Model file for the job. Use its own axes, mm. Give positions to 0.01 mm unless a question says otherwise; leave off trailing zeros. Order: outer loops, then holes, each group sorted by start corner. A loop starts at its lowest first (then second) coordinate and runs counter-clockwise, first axis right, second up. Notation, with made-up numbers: M 40,47 L 87,47 A24 ccw 87,57 Z; hole C 20.25,-31 d9. An arc over 180 degrees is marked long. Return JSON: item names as keys, results as strings. Group by question number.
1. Slice it at B-B on x = 13.5. List the corners of the cut face in (y, z), then the cut area to 3 significant figures.
2. Slice it at A-A on x = -18. List the corners of the cut face in (y, z), then the cut area to 3 significant figures.
3. Pin check, flat tip, straight feed: pin 1 (2 mm diameter, centred on x = -10.5, z = 4.5, fed in from -Y). Stop position of the tip, or through.
4. Wall check: probe 1 along Y at (x, z) = (-15.5, 0); probe 2 along Z at (x, y) = (-8, 12.7); probe 3 along Z at (x, y) = (-22.5, 5.75). Give the ranges that are in metal, low to high. Write a range as [from, to].
5. Two-plate mould, pull along Y, no slides. Class faces 1 (the face through (0, 25.4, 0)), 2 (the face through (0, 13, 12.7)), 3 (the face through (-6, 4, 2)), 4 (the face through (7.232, 1.229, 0.805)): released by +Y, released by -Y, zero draft, split by the parting line, or undercut.
from build123d import *

# Parameters (mm, degrees)
SKETCH1_W                         = 50.8
SKETCH1_H                         = 25.4
BOSS_EXTRUDE1_DEPTH               = 25.4
PIPE_TAP_DRILL_FOR_1_2_TAP1_D     = 17.8562
PIPE_TAP_DRILL_FOR_1_2_TAP1_DEPTH = 38.1
PIPE_TAP_DRILL_FOR_1_2_TAP1_TIP   = 5.364543693


with BuildPart() as part:
    # Sketch1 → Boss-Extrude1 (new body)
    with BuildSketch(Plane(origin=(0, 0, 0), x_dir=(1, 0, 0), z_dir=(0, 1, 0))):
        Rectangle(SKETCH1_W, SKETCH1_H)
    extrude(amount=BOSS_EXTRUDE1_DEPTH)

    # Pipe Tap Drill for 1/2 Tap1
    with Locations(Plane.ZY.offset(25.4)):
        with Locations((0, 12.7)):
            Hole(PIPE_TAP_DRILL_FOR_1_2_TAP1_D / 2, depth=PIPE_TAP_DRILL_FOR_1_2_TAP1_DEPTH)
            with Locations((0, 0, -(PIPE_TAP_DRILL_FOR_1_2_TAP1_DEPTH + PIPE_TAP_DRILL_FOR_1_2_TAP1_TIP / 2))):  # 118° drill point
                Cone(0, PIPE_TAP_DRILL_FOR_1_2_TAP1_D / 2, PIPE_TAP_DRILL_FOR_1_2_TAP1_TIP, mode=Mode.SUBTRACT)

    # Sketch5 → Cut-Revolve2 (revolve, cut)
    with BuildSketch(Plane.XY):
        Polygon((-12.7, -10.766878787), (-9.352189393, -14.114689393), (11.954399011, 7.191899011), (11.1125, 8.033798023), (-0.841899011, -3.920600989), align=None)
    revolve(axis=Axis((-9.352189393, -14.114689393, 0), (0.707106781, 0.707106781, 0)), mode=Mode.SUBTRACT)


solid = part.part
Result:
{
 "1": {"outline": "M 0,-12.7 L 25.4,-12.7 L 25.4,12.7 L 0,12.7 Z; hole C 12.7,0 d15.19", "area": "464 mm2"},
 "2": {"outline": "M 0,-12.7 L 25.4,-12.7 L 25.4,12.7 L 0,12.7 Z; hole C 12.7,0 d17.86", "area": "395 mm2"},
 "3": {"pin 1": "stops at y = 0"},
 "4": {"probe 1": "y = [0, 3.77], [21.63, 25.4]", "probe 2": "z = [-12.7, -8.93], [8.93, 12.7]", "probe 3": "z = [-12.7, -5.6], [5.6, 12.7]"},
 "5": {"face 1": "released by +Y", "face 2": "zero draft", "face 3": "undercut", "face 4": "undercut"}
}
